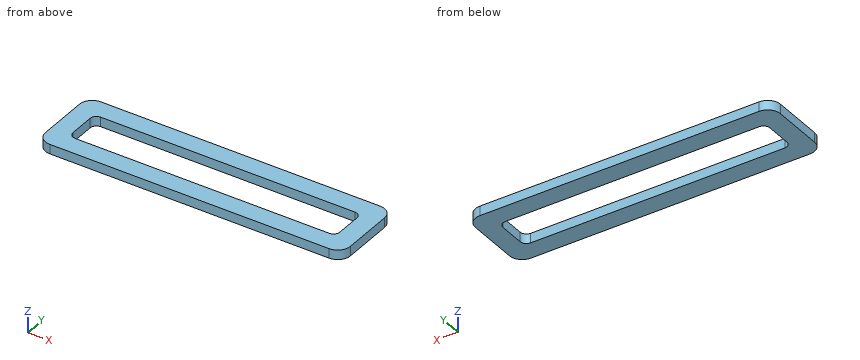
```python
from build123d import *

# Parameters (mm, degrees)
SKETCH1_W           = 304.8
SKETCH1_H           = 76.2
SKETCH1_W_2         = 266.7
SKETCH1_H_2         = 38.1
BOSS_EXTRUDE1_DEPTH = 9.525
FILLET1_R           = 12.7
FILLET2_R           = 6.35


with BuildPart() as part:
    # Sketch1 → Boss-Extrude1 (new body)
    with BuildSketch(Plane.XY):
        Rectangle(SKETCH1_W, SKETCH1_H)
        Rectangle(SKETCH1_W_2, SKETCH1_H_2, mode=Mode.SUBTRACT)
    extrude(amount=BOSS_EXTRUDE1_DEPTH)

    # Fillet1
    fillet1_edges = [part.edges().sort_by_distance(p)[0] for p in [
        (152.4, -38.1, 4.7625),
        (-152.4, -38.1, 4.7625),
        (-152.4, 38.1, 4.7625),
        (152.4, 38.1, 4.7625),
    ]]
    fillet(fillet1_edges, radius=FILLET1_R)

    # Fillet2
    fillet2_edges = [part.edges().sort_by_distance(p)[0] for p in [
        (133.35, -19.05, 4.7625),
        (133.35, 19.05, 4.7625),
        (-133.35, 19.05, 4.7625),
        (-133.35, -19.05, 4.7625),
    ]]
    fillet(fillet2_edges, radius=FILLET2_R)


solid = part.part
```
Could you check a few things on this model? Use its own coordinates, in mm. Coordinates: 2 decimals unless noted, no trailing zeros. Write each loop counter-clockwise with the first axis right and the second up, starting at its lowest first coordinate (ties: lowest second). Pieces come first, ordered by that corner, then holes. Notation, with made-up numbers: (27, 7.5) -> (73, 7.5) arc R29 ccw to (73, 31.5) -> close; hole circle Ø1 at (-23.5, -13). An arc over 180 degrees is marked (long way). One line per question, with ' | ' between items. Start each with the question number.
1. If we section it at B-B (x = -36): Please give me the cut outline in (y, z) (3 decimals).
2. Please list where these lines run through material, in increasing order: line 1 along Y through (x, z) = (53, 6.25); line 2 along X through (y, z) = (-3.5, 6); line 3 along X through (y, z) = (26.5, 7.75).
3. Will this pin go through, and if not, where does the flat tip stop? P1, Ø4, axis at x = 116, y = 17.5, coming from the -Z side.
4. If we section it at C-C (z = 5.5): Please give me the cut outline in (x, y), and give its area (3 significant figures).
5. If we section it at A-A (y = 3.5): Please give me the cut outline in (x, z) (3 decimals).
Return value:
1) outline: (-38.1, 0) -> (-19.05, 0) -> (-19.05, 9.525) -> (-38.1, 9.525) -> close; (19.05, 0) -> (38.1, 0) -> (38.1, 9.525) -> (19.05, 9.525) -> close
2) line 1: y = -38.1 to -19.05, 19.05 to 38.1 | line 2: x = -152.4 to -133.35, 133.35 to 152.4 | line 3: x = -152.35 to 152.35
3) P1: stops at z = 0
4) outline: (-152.4, -25.4) arc R12.7 ccw to (-139.7, -38.1) -> (139.7, -38.1) arc R12.7 ccw to (152.4, -25.4) -> (152.4, 25.4) arc R12.7 ccw to (139.7, 38.1) -> (-139.7, 38.1) arc R12.7 ccw to (-152.4, 25.4) -> close; hole (-133.35, -12.7) arc R6.35 ccw to (-127, -19.05) -> (127, -19.05) arc R6.35 ccw to (133.35, -12.7) -> (133.35, 12.7) arc R6.35 ccw to (127, 19.05) -> (-127, 19.05) arc R6.35 ccw to (-133.35, 12.7) -> close | area: 13,000 mm²
5) outline: (-152.4, 0) -> (-133.35, 0) -> (-133.35, 9.525) -> (-152.4, 9.525) -> close; (133.35, 0) -> (152.4, 0) -> (152.4, 9.525) -> (133.35, 9.525) -> close
